Verification items for the finished model (mm, model axes). A direction names the side the tool comes from. Coordinates: 2 decimals unless noted, no trailing zeros. Write each loop counter-clockwise with the first axis right and the second up, starting at its lowest first coordinate (ties: lowest second). Pieces come first, ordered by that corner, then holes. Notation, with made-up numbers: (23, 56) -> (79, 56) arc R15 ccw to (79, 76) -> close; hole circle Ø8 at (37.5, 41.5). An arc over 180 degrees is marked (long way). Write each question's results on one line, items separated by ' | '. Start each with the question number.
from build123d import *

# Parameters (mm, degrees)
SKETCH2_R           = 60
BOSS_EXTRUDE1_DEPTH = 3
SKETCH3_R           = 63
SKETCH3_R_2         = 60
BOSS_EXTRUDE2_DEPTH = 10


with BuildPart() as part:
    # Sketch2 → Boss-Extrude1 (new body)
    with BuildSketch(Plane(origin=(0, 0, 0), x_dir=(1, 0, 0), z_dir=(0, 1, 0))):
        with BuildLine():
            Line((0, -85), (103.666002653, -85))
            Line((103.666002653, -85), (103.666002653, -15))
            Line((103.666002653, -15), (83.666002653, -15))
            ThreePointArc((83.666002653, -15), (-54.543560573, 65.192024052), (0, -85))
        make_face()
        Circle(SKETCH2_R, mode=Mode.SUBTRACT)
    extrude(amount=BOSS_EXTRUDE1_DEPTH)

    # Sketch3 → Boss-Extrude2 (add)
    with BuildSketch(Plane(origin=(0, 3, 0), x_dir=(1, 0, 0), z_dir=(0, 1, 0))):
        Circle(SKETCH3_R)
        Circle(SKETCH3_R_2, mode=Mode.SUBTRACT)
    extrude(amount=BOSS_EXTRUDE2_DEPTH)


solid = part.part
1. Mould release check, pull along X, two halves, no side actions. Record for faces 1 (the cylindrical face through (-52.28, 1.48, -67.02)), 2 (the flat face through (56, 13, 23)), 3 (the cylindrical face through (-59.94, 6.41, -2.64)): +X half, -X half, draft (parallel to the pull), parting line (faces both ways), or undercut.
2. Material ranges on probe 1 along X at (y, z) = (8.5, 0); probe 2 along X at (y, z) = (2.5, 0), recorded low to high. Write a range as from..to.
3. Sectioned sample at C-C on y = 6.5. Record the cut outline in (x, z), plus the area to 3 significant figures.
4. Tool access check on faces 4 (the flat face through (50, 0, 37)), 5 (the flat face through (71, 3, 18)). Record the directions out of +Z, -Z, +X, -X, +Y, -Y that give a thin tool (end or side, any length) a straight path to the whole face; none if there is none.
5. Depth check by flat-ended pin: pin 1 Ø5 at (y, z) = (11.5, 48) entering from +X; pin 2 Ø3 at (y, z) = (6.5, -19.5) entering from +X; pin 3 Ø1 at (x, y) = (45.5, 7) entering from +Z. Enter the tip coordinate at first touch or a pass-through.
6. Sectioned sample at A-A on z = 0. Record the cut outline in (x, y), plus the area to 3 significant figures.
7. Sectioned sample at B-B on x = -15. Record the cut outline in (y, z), plus the area to 3 significant figures.
8. Sectioned sample at D-D on z = -69.5. Record the cut outline in (x, y).
Computed values:
1) face 1: parting line | face 2: draft | face 3: undercut
2) probe 1: x = -63..-60, 60..63 | probe 2: x = -85..-60, 60..85
3) outline: circle Ø126 at (0, 0); hole circle Ø120 at (0, 0) | area: 1,160 mm^2
4) face 4: +Z, -Z, +X, -X, -Y | face 5: +Y
5) pin 1: stops at x = 43.57 | pin 2: stops at x = 60.37 | pin 3: stops at z = 44.09
6) outline: (-85, 0) -> (-60, 0) -> (-60, 13) -> (-63, 13) -> (-63, 3) -> (-85, 3) -> close; (60, 0) -> (85, 0) -> (85, 3) -> (63, 3) -> (63, 13) -> (60, 13) -> close | area: 210 mm^2
7) outline: (0, -83.67) -> (3, -83.67) -> (3, -61.19) -> (13, -61.19) -> (13, -58.09) -> (0, -58.09) -> close; (0, 58.09) -> (13, 58.09) -> (13, 61.19) -> (3, 61.19) -> (3, 83.67) -> (0, 83.67) -> close | area: 215 mm^2
8) outline: (-48.94, 0) -> (48.94, 0) -> (48.94, 3) -> (-48.94, 3) -> close
